The model under review builds one solid part; all positions refer to its coordinate system, in mm. A direction names the side the tool comes from. Coordinates: 2 decimals unless noted, no trailing zeros. Loops run counter-clockwise (first coordinate to the right, second up) from the corner with the lowest first, then second, coordinate; pieces in that order, holes last. Notation, with made-up numbers: M -11.75,20.25 L 10.25,20.25 A25 cw 10.25,57.25 Z; hole C 25.25,9.25 d10. An arc over 180 degrees is marked long. Return JSON: item names as keys, results as strings.
```python
from build123d import *

# Parameters (mm, degrees)
SKETCH1_R           = 4.9
BOSS_EXTRUDE1_DEPTH = 50
BOSS_EXTRUDE2_DEPTH = 5


with BuildPart() as part:
    # Sketch1 → Boss-Extrude1 (new body)
    with BuildSketch(Plane(origin=(0, 0, 0), x_dir=(1, 0, 0), z_dir=(0, 1, 0))):
        with Locations(Location((0, 0, 0), (0, 0, 270))):
            Circle(SKETCH1_R)
    extrude(amount=BOSS_EXTRUDE1_DEPTH)

    # Sketch2 → Boss-Extrude2 (add)
    with BuildSketch(Plane(origin=(0, 50, 0), x_dir=(1, 0, 0), z_dir=(0, 1, 0))):
        with BuildLine():
            Line((0, 4.9), (-50, 4.9))
            Line((-50, 4.9), (-50, -5))
            Line((-50, -5), (0, -5))
            ThreePointArc((0, -5), (5.705336799, -0.05), (0, 4.9))
        make_face()
    extrude(amount=BOSS_EXTRUDE2_DEPTH)


solid = part.part
```
1. Add section C-C on y = 30.5. Give the boundary of the cut face in (x, z).
Check values:
{"outline": "C 0,0 d9.8"}
2. Insertion check: pin 1 Ø5.5 at (x, y) = (-36, 51.5) entering from +Z; pin 2 Ø5 at (x, z) = (-17, -1) entering from -Y; pin 3 Ø2 at (y, z) = (27.5, 2.5) entering from -X. Each pin has a flat end and moves straight along its axis. Give the tip position at first contact, or say it passes through.
Check values:
{"pin 1": "z = 5", "pin 2": "y = 50", "pin 3": "x = -4.66"}
3. Add section A-A on z = -3. Give the boundary of the cut face in (x, y).
Check values:
{"outline": "M -50,50 L -3.87,50 L -3.87,0 L 3.87,0 L 3.87,50 L 4.67,50 L 4.67,55 L -50,55 Z"}
4. Add section D-D on z = 4. Give the boundary of the cut face in (x, y).
Check values:
{"outline": "M -50,50 L -2.83,50 L -2.83,0 L 2.83,0 L 2.83,50 L 3.77,50 L 3.77,55 L -50,55 Z"}
5. Machinability: for faces 1 (the face through (-25, 52, 5)), 2 (the face through (1.472, 24.65, 4.674)), 3 (the face through (-50, 52, 0)), 4 (the face through (-23, 55, 0)), 5 (the face through (-25, 52, -4.9)), which of the approach directions +Z, -Z, +X, -X, +Y, -Y give a long, thin tool a straight path to every point of the face, cutting with its end or side? Answer none if there is none.
Check values:
{"face 1": "+Z, -X, +Y, -Y", "face 2": "-Y", "face 3": "+Z, -Z, -X, +Y, -Y", "face 4": "+Z, -Z, +X, -X, +Y", "face 5": "-Z, -X, +Y, -Y"}
6. Add section B-B on x = -17. Give the boundary of the cut face in (y, z), plus the area to 3 significant figures.
Check values:
{"outline": "M 50,-4.9 L 55,-4.9 L 55,5 L 50,5 Z", "area": "49.5 mm²"}
7. To check wall thickness, follow line 1 (Y direction, x = -41, z = 0.25); line 2 (X direction, y = 14.5, z = 0); line 3 (X direction, y = 30, z = -4). State the ranges of each line that lie inside material, in increasing order.
Check values:
{"line 1": "50 to 55", "line 2": "-4.9 to 4.9", "line 3": "-2.83 to 2.83"}
